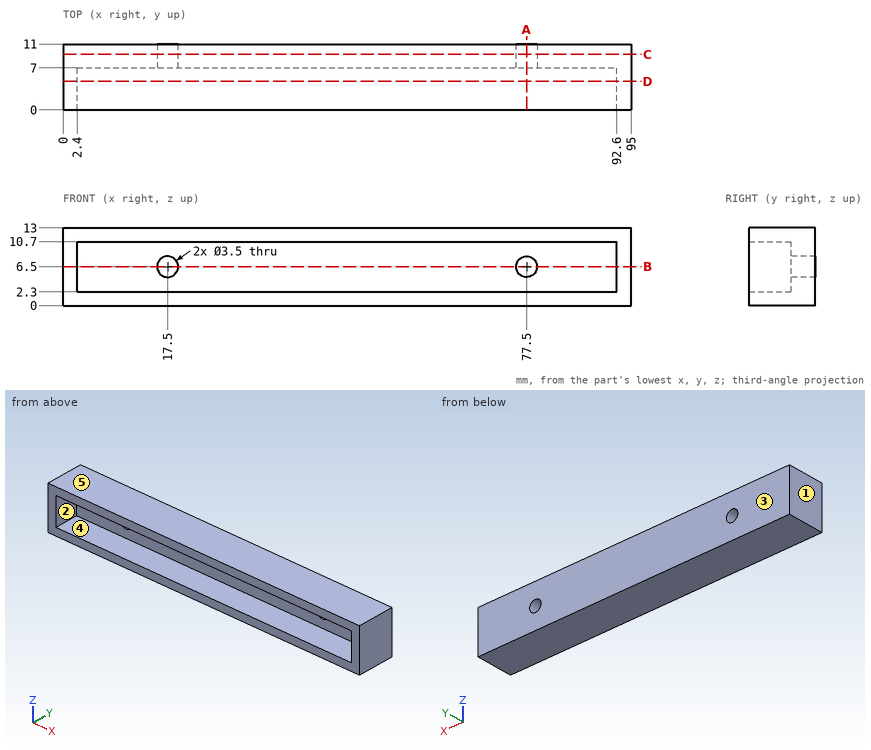
Job drawing, mm, ordinate dimensions from the low corner. One solid piece. A direction names the side the tool comes from. Give positions to 0.01 mm unless a question says otherwise; leave off trailing zeros. Loops run counter-clockwise (first coordinate to the right, second up) from the corner with the lowest first, then second, coordinate; pieces in that order, holes last.
Item 1: Drill centre lines: line 1 (Z direction, x = 69, y = 0.5); line 2 (X direction, y = 5.75, z = 2.75); line 3 (Z direction, x = 17.5, y = 10). Where is each one in solid material? Low to high.
Answers follow:
line 1: z = 0 to 2.3, 10.7 to 13
line 2: x = 0 to 2.4, 92.6 to 95
line 3: z = 0 to 4.75, 8.25 to 13
Item 2: Flat gauge pins, fed straight in: pin 1 (4.5 mm diameter, centred on x = 77.5, z = 6.5, fed in from -Y); pin 2 (3 mm diameter, centred on x = 17.5, z = 6.5, fed in from +Y). Where does each tip first touch, or does it go through?
Answers follow:
pin 1: stops at y = 7
pin 2: passes through
Item 3: Pull direction Z, two halves, no side cores. Call the marked faces 3, 4 and 5: released by +Z, released by -Z, zero draft, split by the parting line, or undercut.
Answers follow:
face 3: zero draft
face 4: undercut
face 5: released by +Z
Item 4: Slice it at D-D, the plane y = 4.75. List the corners of the cut face in (x, z).
Answers follow:
outline: (0, 0) - (95, 0) - (95, 13) - (0, 13) - close; hole (2.4, 2.3) - (92.6, 2.3) - (92.6, 10.7) - (2.4, 10.7) - close
Item 5: Slice it at A-A, the plane x = 77.5. List the corners of the cut face in (y, z).
Answers follow:
outline: (0, 0) - (11, 0) - (11, 4.75) - (7, 4.75) - (7, 2.3) - (0, 2.3) - close; (0, 10.7) - (7, 10.7) - (7, 8.25) - (11, 8.25) - (11, 13) - (0, 13) - close
Item 6: Which spindle directions (+Z, -Z, +X, -X, +Y, -Y) get a long thin tool onto all of the face, cutting with end or side? Do the marked faces 1 and 2. Say none if no direction does.
Answers follow:
face 1: +Z, -Z, -X, +Y, -Y
face 2: -Y
Item 7: Slice it at C-C, the plane y = 9.25. List the corners of the cut face in (x, z), and give its area (3 significant figures).
Answers follow:
outline: (0, 0) - (95, 0) - (95, 13) - (0, 13) - close; hole circle Ø3.5 at (17.5, 6.5); hole circle Ø3.5 at (77.5, 6.5)
area: 1,220 mm2
Item 8: Slice it at B-B, the plane z = 6.5. List the corners of the cut face in (x, y).
Answers follow:
outline: (0, 0) - (2.4, 0) - (2.4, 7) - (15.75, 7) - (15.75, 11) - (0, 11) - close; (19.25, 7) - (75.75, 7) - (75.75, 11) - (19.25, 11) - close; (79.25, 7) - (92.6, 7) - (92.6, 0) - (95, 0) - (95, 11) - (79.25, 11) - close
